Geometry check sheet. Reference: the model listing, model coordinates, mm. A direction names the side the tool comes from. Give positions to 0.01 mm unless a question says otherwise; leave off trailing zeros. Order: outer loops, then holes, each group sorted by start corner. A loop starts at its lowest first (then second) coordinate and runs counter-clockwise, first axis right, second up. Notation, with made-up numbers: M 21.25,16 L 30.25,16 A14 ccw 30.25,20 Z; hole C -33.5,-7 d11. An arc over 180 degrees is marked long. Answer as a JSON object with one key per item and string values. Group by question number.
Autodesk Inventor part; units mm, degrees
ref_plane "YZ Plane" through (0, 0, 0) normal (1, 0, 0) x (0, 1, 0)
ref_plane "XZ Plane" through (0, 0, 0) normal (0, 1, 0) x (-1, 0, 0)
ref_plane "XY Plane" through (0, 0, 0) normal (0, 0, 1) x (1, 0, 0)
sketch "Sketch1" plane through (0, 0, 0) normal (0, 1, 0) x (-1, 0, 0)
  line L0 (90, -50) -> (-90, -50)
  line L1 (-90, -50) -> (-90, 50)
  line L2 (-90, 50) -> (90, 50)
  line L3 (90, 50) -> (90, -50)
  line L4 (0, 0) -> (0, -16.1308) construction
  line L5 (0, 0) -> (18.4922, 0) construction
  dimension "d1" = 100
  dimension "d2" = 180
extrude "Extrusion1" add sketch "Sketch1" along normal blind 2.2
sketch "Sketch2" plane through (0, 2.2, 0) normal (0, 1, 0) x (1, 0, 0)
  line L0 (-90, -50) -> (90, -50)
  line L1 (90, -50) -> (90, 50)
  line L2 (90, -50) -> (90, -30)
  line L3 (90, -30) -> (55.6, -30)
  line L4 (55.6, -30) -> (55.6, -50)
  line L5 (55.6, -50) -> (90, -50)
  line L6 (90, -40) -> (55.6, -40) construction
  circle A0 centre (78.8, -40) radius 2.15
  circle A1 centre (72.8, -40) radius 2.15
  circle A2 centre (66.8, -40) radius 2.15
  line L7 (72.8, -40) -> (72.8, -30) construction
  circle A3 centre (72.8, -34) radius 2.15
  circle A4 centre (72.8, -46) radius 2.15
  circle A5 centre (72.8, -40) radius 2.15
  line L8 (0, 0) -> (96.2626, 0) construction
  line L9 (90, 50) -> (90, 30)
  line L10 (90, 30) -> (55.6, 30)
  line L11 (55.6, 30) -> (55.6, 50)
  line L12 (55.6, 50) -> (90, 50)
  line L13 (90, 40) -> (55.6, 40) construction
  circle A6 centre (78.8, 40) radius 2.15
  circle A7 centre (72.8, 40) radius 2.15
  circle A8 centre (66.8, 40) radius 2.15
  line L14 (72.8, 40) -> (72.8, 30) construction
  circle A9 centre (72.8, 34) radius 2.15
  circle A10 centre (72.8, 46) radius 2.15
  circle A11 centre (72.8, 40) radius 2.15
  line L15 (90, 50) -> (-90, 50)
  line L16 (-90, 50) -> (-90, -50)
  line L17 (-48, 40) -> (-72, 40)
  line L18 (-72, 40) -> (-72, 50)
  line L19 (-72, 50) -> (-48, 50)
  line L20 (-48, 50) -> (-48, 40)
  line L21 (-74.3246, 46.5) -> (-4.1674, 46.5) construction
  line L22 (-60, 53.3324) -> (-60, 32.9187) construction
  circle A12 centre (-60, 37.5) radius 2.15
  line L23 (-68.3246, 46.5) -> (1.8326, 46.5) construction
  circle A13 centre (-54, 37.5) radius 2.15
  circle A14 centre (-66, 37.5) radius 2.15
  line L24 (-8.0003, 43.25) -> (-83.9137, 43.25) construction
  circle A15 centre (-78, 43.25) radius 2.15
  circle A16 centre (-84, 43.25) radius 2.15
  circle A17 centre (-42, 43.25) radius 2.15
  circle A18 centre (-36, 43.25) radius 2.15
  line L25 (-48, -40) -> (-72, -40)
  line L26 (-72, -40) -> (-72, -50)
  line L27 (-72, -50) -> (-48, -50)
  line L28 (-48, -50) -> (-48, -40)
  line L29 (-74.3246, -46.5) -> (-4.1674, -46.5) construction
  line L30 (-60, -53.3324) -> (-60, -32.9187) construction
  circle A19 centre (-60, -37.5) radius 2.15
  circle A20 centre (-54, -37.5) radius 2.15
  circle A21 centre (-66, -37.5) radius 2.15
  line L31 (-8.0003, -43.25) -> (-83.9137, -43.25) construction
  circle A22 centre (-78, -43.25) radius 2.15
  circle A23 centre (-84, -43.25) radius 2.15
  circle A24 centre (-36, -43.25) radius 2.15
  circle A25 centre (-42, -43.25) radius 2.15
  circle A26 centre (-60, 37.5) radius 2.5 construction
  dimension "d13" = 20
  dimension "d14" = 34.4
  dimension "d15" = 4.3
  dimension "d16" = 6
  dimension "d17" = 6
  dimension "d18" = 6
  dimension "d27" = 24
  dimension "d28" = 10
  dimension "d29" = 18
  dimension "d31" = 4.3
  dimension "d34" = 6
  dimension "d41" = 6
  dimension "d46" = 6.5
  dimension "d48" = 4.3
  dimension "d49" = 6
  dimension "d52" = 6
  dimension "d60" = 5
extrude "Holes" cut sketch "Sketch2" against normal through all contours A0 | A1 | A2 | A3 | A4 | A6 | A7 | A8 | A9 | A10 | A12 | A13 | A14 | A15 | A16 | A17 | A18 | A19 | A20 | A21 | A22 | A23 | A24 | A25
sketch "Sketch3" plane through (0, 2.2, 0) normal (0, 1, 0) x (1, 0, 0)
  line L0 (33.5, 13.5) -> (-33.5, 13.5) construction
  line L1 (-33.5, 13.5) -> (-33.5, -13.5) construction
  line L2 (-33.5, -13.5) -> (33.5, -13.5) construction
  line L3 (33.5, -13.5) -> (33.5, 13.5) construction
  line L4 (0, 0) -> (39.98, 0) construction
  line L5 (0, 0) -> (0, 21.0122) construction
  circle A0 centre (30, 9) radius 2.15
  circle A1 centre (30, -9) radius 2.15
  circle A2 centre (-30, 9) radius 2.15
  circle A3 centre (-30, -9) radius 2.15
  line L6 (33.5, 7.5) -> (43.5, 7.5)
  line L7 (43.5, 7.5) -> (43.5, -7.5)
  line L8 (43.5, -7.5) -> (33.5, -7.5)
  line L9 (33.5, -7.5) -> (33.5, 7.5)
  dimension "d61" = 67
  dimension "d62" = 27
  dimension "d63" = 4.3
  dimension "d64" = 3.5
  dimension "d65" = 4.5
  dimension "d68" = 10
  dimension "d69" = 15
extrude "Extrusion4" cut sketch "Sketch3" against normal through all
fillet "Fillet1" radius 2 4 edges at (33.5, 1.1, -7.5) (43.5, 1.1, -7.5) (43.5, 1.1, 7.5) (33.5, 1.1, 7.5)
ref_plane "Work Plane1" through (0, 0, 50) normal (1, 0, 0) x (0, 0, -1)
split "Split1" plane through (0, 0, 50) removes the side toward (-1, 0, 0)
sketch "Sketch4" plane through (0, 2.2, 0) normal (0, 1, 0) x (1, 0, 0)
  line L0 (0, 50) -> (0, -50)
  line L1 (0, -50) -> (90, -50)
  line L2 (0, 50) -> (5, 50)
  line L3 (5, 50) -> (5, -50)
  line L4 (5, -50) -> (0, -50)
  line L5 (0, -50) -> (0, 50)
  point P0 (0, 0)
  dimension "d71" = 5
extrude "Extrusion5" add sketch "Sketch4" along normal blind 2.2
sketch "Sketch6" plane through (0, 0, -50) normal (-1, 0, 0) x (0, 0, 1)
  line L0 (100, 4.4) -> (100, 0)
  line L1 (0, 4.4) -> (100, 4.4)
  line L2 (0, 4.4) -> (100, 4.4)
  line L3 (100, 4.4) -> (100, 2.2)
  line L4 (100, 2.2) -> (0, 2.2)
  line L5 (0, 2.2) -> (0, 4.4)
  point P0 (50, 0)
extrude "Extrusion6" add sketch "Sketch6" along normal blind 10
sketch "Sketch7" plane through (0, 4.4, 0) normal (0, 1, 0) x (1, 0, 0)
  line L0 (5, -50) -> (-10, -50)
  line L1 (5, 50) -> (-10, 50)
  line L2 (-10, 50) -> (-5, 50) construction
  line L3 (-5, 50) -> (-5, -50) construction
  line L4 (-5, -50) -> (-10, -50) construction
  line L5 (-10, -50) -> (-10, 50) construction
  line L6 (0, 0) -> (-18.3669, 0) construction
  circle A0 centre (-5, 37.5) radius 1.3
  circle A1 centre (-5, 25) radius 1.3
  circle A2 centre (-5, -37.5) radius 1.3
  circle A3 centre (-5, -25) radius 1.3
  dimension "d76" = 5
  dimension "d77" = 2.6
  dimension "d78" = 12.5
  dimension "d81" = 12.5
extrude "Extrusion7" cut sketch "Sketch7" against normal through all
fillet "Fillet2" radius 2 2 edges at (-10, 4.4, 0) (5, 4.4, 0)
equation "\"d1\" = BodyWidth"
equation "\"d2\" = BodyLength"
equation "\"d3\" = Depth"
equation "\"d15\" = Holes"
equation "\"d27\" = MotorWidth"
equation "\"d31\" = Holes"
equation "\"d57\" = Depth"
equation "\"d72\" = Depth"
equation "\"d78\" = 0.125 * BodyWidth"
equation "\"d81\" = 0.125 * BodyWidth"
equation "\"BodyWidth\" = 100"
equation "\"BodyLength\" = 180"
equation "\"Holes\" = 4.3"
equation "\"Depth\" = 2.2"
equation "\"d20\" = 4.3"
equation "\"MotorWidth\" = 24"
properties part number "BodyBack"
1. Release check for a two-part mould opening along Z. For faces 4 (the flat face through (-2, 4.4, -1)), 5 (the cylindrical face through (66.52, 1.12, 37.87)), 6 (the flat face through (41, 1, -50)) record: released by +Z, released by -Z, zero draft, split by the parting line, or undercut.
2. Cross-section at A-A (x = 78.8). Record the cut outline in (y, z).
3. Cross-section at D-D (x = -5). Record the cut outline in (y, z), and give its area (3 significant figures).
4. Cross-section at B-B (z = -9). Record the cut outline in (x, y).
5. Cross-section at C-C (y = 1.3). State how many separate pieces and enclosed holes the cut face has, and give its area (3 significant figures).
6. Depth check by flat-ended pin: pin 1 (1 mm diameter, centred on x = 80, z = 3.5, fed in from +Y); pin 2 (3 mm diameter, centred on x = -5, z = -37.5, fed in from -Y); pin 3 (4 mm diameter, centred on x = 72.8, z = -40, fed in from +Y); pin 4 (1.1 mm diameter, centred on y = 1, z = -1, fed in from -X). Enter the tip coordinate at first touch or a pass-through.
7. Access from +Z, -Z, +X, -X, +Y, -Y to the whole of each face (thin tool, end or side, straight path). Record for faces 1 (the flat face through (90, 1, -1)), 2 (the flat face through (0, 1, -1)), 3 (the flat face through (38, 1, -7.5)).
8. Thickness scan on line 1 along Z through (x, y) = (30, 1.55); line 2 along X through (y, z) = (0.8, -40); line 3 along Z through (x, y) = (-4, 2.5). Record the ranges inside material, lowest first. Write a range as [from, to].
Report:
{
 "1": {"face 4": "zero draft", "face 5": "undercut", "face 6": "released by -Z"},
 "2": {"outline": "M 0,-50 L 2.2,-50 L 2.2,-42.15 L 0,-42.15 Z; M 0,-37.85 L 2.2,-37.85 L 2.2,37.85 L 0,37.85 Z; M 0,42.15 L 2.2,42.15 L 2.2,50 L 0,50 Z"},
 "3": {"outline": "M 2.2,-50 L 4.4,-50 L 4.4,-38.8 L 2.2,-38.8 Z; M 2.2,-36.2 L 4.4,-36.2 L 4.4,-26.3 L 2.2,-26.3 Z; M 2.2,-23.7 L 4.4,-23.7 L 4.4,23.7 L 2.2,23.7 Z; M 2.2,26.3 L 4.4,26.3 L 4.4,36.2 L 2.2,36.2 Z; M 2.2,38.8 L 4.4,38.8 L 4.4,50 L 2.2,50 Z", "area": "197 mm2"},
 "4": {"outline": "M -10,2.2 L 0,2.2 L 0,0 L 27.85,0 L 27.85,2.2 L 5,2.2 L 5,2.4 A2 ccw 3,4.4 L -8,4.4 A2 ccw -10,2.4 Z; M 32.15,0 L 90,0 L 90,2.2 L 32.15,2.2 Z"},
 "5": {"separate pieces": "1", "enclosed holes": "13", "area": "8,680 mm2"},
 "6": {"pin 1": "stops at y = 2.2", "pin 2": "stops at y = 2.2", "pin 3": "passes through", "pin 4": "stops at x = 0"},
 "7": {"face 1": "+Z, -Z, +X, +Y, -Y", "face 2": "+Z, -Z, -X, -Y", "face 3": "+Y, -Y"},
 "8": {"line 1": "z = [-50, -11.15], [-6.85, 6.85], [11.15, 50]", "line 2": "x = [0, 64.65], [68.95, 70.65], [74.95, 76.65], [80.95, 90]", "line 3": "z = [-50, -38.33], [-36.67, -25.83], [-24.17, 24.17], [25.83, 36.67], [38.33, 50]"}
}
